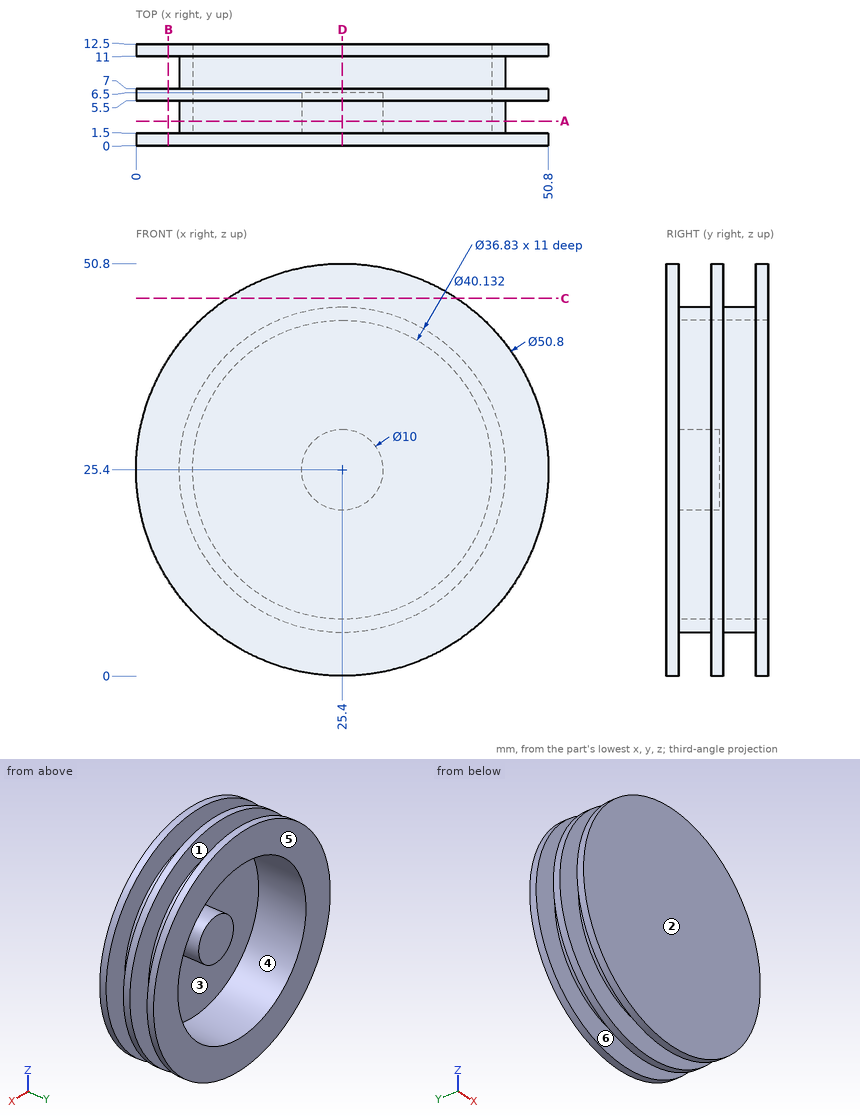
Design review of the part shown in the three views and the two pictorial views. Dimensions are in mm from the part's minimum x, y and z. A direction names the side the tool comes from. Round coordinates to 2 decimals unless told otherwise and drop trailing zeros. Write each loop counter-clockwise with the first axis right and the second up, starting at its lowest first coordinate (ties: lowest second). Pieces come first, ordered by that corner, then holes.
Item 1: Consider section D-D on x = 25.4. Give the boundary of the cut face in (y, z) (3 decimals).
Item 2: For pin 1 Ø5 at (x, z) = (38, 16.5) entering from +Y; pin 2 Ø6 at (x, y) = (14, 1.5) entering from +Z; pin 3 Ø11 at (x, z) = (25.5, 24) entering from +Y, all flat-tipped, find the tip position at first contact; note any pin that passes through.
Item 3: Consider section A-A on y = 3. Give the boundary of the cut face in (x, z) (3 decimals).
Item 4: Draft analysis for pull direction Y (two halves, no side actions). For the marked faces 4, 5 and 6, state which applies: released by +Y, released by -Y, zero draft, split by the parting line, or undercut.
Item 5: For the marked faces 1, 2 and 3, list the 3-axis set-ups (+Z, -Z, +X, -X, +Y, -Y) from which the entire face can be reached by the end or side of a thin tool; tool diameter is ignored.
Item 6: Consider section C-C on z = 46.5. Give the boundary of the cut face in (x, y).
Item 7: Wall thickness on L1, parallel to Y at x = 36, z = 3; L2, parallel to X at y = 4.5, z = 25.4 (3 decimals); L3, parallel to X at y = 6, z = 25.4 (3 decimals): over which ranges is each line inside the solid? List them lowest first.
Item 8: Consider section B-B on x = 4. Give the boundary of the cut face in (y, z), and give its area (3 significant figures).
Check values:
1. outline: (0, 0) - (1.5, 0) - (1.5, 5.334) - (5.5, 5.334) - (5.5, 0) - (7, 0) - (7, 5.334) - (11, 5.334) - (11, 0) - (12.5, 0) - (12.5, 6.985) - (1.5, 6.985) - (1.5, 20.4) - (6.5, 20.4) - (6.5, 30.4) - (1.5, 30.4) - (1.5, 43.815) - (12.5, 43.815) - (12.5, 50.8) - (11, 50.8) - (11, 45.466) - (7, 45.466) - (7, 50.8) - (5.5, 50.8) - (5.5, 45.466) - (1.5, 45.466) - (1.5, 50.8) - (0, 50.8) - close
2. pin 1: stops at y = 1.5
2. pin 2: stops at z = 49.37
2. pin 3: stops at y = 6.5
3. outline: circle Ø40.132 at (25.4, 25.4); circle Ø10 at (25.4, 25.4); hole circle Ø36.83 at (25.4, 25.4)
4. face 4: zero draft
4. face 5: released by +Y
4. face 6: undercut
5. face 1: none
5. face 2: +Z, -Z, +X, -X, -Y
5. face 3: +Y
6. outline: (11.26, 0) - (39.54, 0) - (39.54, 1.5) - (11.26, 1.5) - close; (11.26, 5.5) - (39.54, 5.5) - (39.54, 7) - (11.26, 7) - close; (11.26, 11) - (39.54, 11) - (39.54, 12.5) - (11.26, 12.5) - close
7. L1: y = 0 to 1.5, 5.5 to 7, 11 to 12.5
7. L2: x = 5.334 to 6.985, 20.4 to 30.4, 43.815 to 45.466
7. L3: x = 0 to 6.985, 20.4 to 30.4, 43.815 to 50.8
8. outline: (0, 11.72) - (1.5, 11.72) - (1.5, 39.08) - (0, 39.08) - close; (5.5, 11.72) - (7, 11.72) - (7, 39.08) - (5.5, 39.08) - close; (11, 11.72) - (12.5, 11.72) - (12.5, 39.08) - (11, 39.08) - close
8. area: 123 mm2
